Part model, mm, in its own coordinate system. Round coordinates to 2 decimals unless told otherwise and drop trailing zeros. Write each loop counter-clockwise with the first axis right and the second up, starting at its lowest first coordinate (ties: lowest second). Pieces come first, ordered by that corner, then holes. Notation, with made-up numbers: M 67.5,82 L 100.5,82 A22 cw 100.5,102 Z; hole C 81,83.25 d1. An arc over 180 degrees is marked long. Use a Markdown table: item, result. Add a question column.
1) Wall check: probe 1 along X at (y, z) = (-150, 0.85); probe 2 along X at (y, z) = (-32.5, 0.7); probe 3 along Y at (x, z) = (47.5, 0.5). Give the ranges that are in metal, low to high.
2) Slice it at C-C on x = -55.5. Write the cut outline in (y, z), plus the area to 3 significant figures.
3) Two-plate mould, pull along X, no slides. Class faces 1 (the face through (-42.88, -78.28, 0.99)), 2 (the face through (25.72, -165.49, 0.99)), 3 (the face through (-58.785, -0.875, 0.986)): released by +X, released by -X, zero draft, split by the parting line, or undercut.
4) Slice it at A-A on y = -145.5. Write the cut outline in (x, z), plus the area to 3 significant figures.
5) Slice it at B-B on z = 0.3. Give the number of separate pieces and of enclosed holes in the cut face, plus the area to 3 significant figures.
6) Drop flat-ended pins along their axis: P1, Ø1, axis at y = 27, z = 0.5, coming from the -X side (3 decimals); P2, Ø1.5, axis at x = 59.22, y = 46.85, coming from the -Z side. Give the stop position or say it passes through.
```python
from build123d import *

# Parameters (mm, degrees)
BOSS_EXTRUDE1_DEPTH = 2
SKETCH3_R           = 1.25
F_45_DEGREES_DEPTH  = 188.552659272
SKETCH4_R           = 1.5
CUT_EXTRUDE2_DEPTH  = 188.552659272
FILLET1_R           = 5
FILLET2_R           = 5
FILLET3_R           = 5
FILLET4_R           = 5
FILLET5_R           = 5
FILLET6_R           = 5
FILLET7_R           = 5
FILLET8_R           = 5
FILLET9_R           = 5
FILLET10_R          = 5
FILLET11_R          = 5
FILLET12_R          = 5


with BuildPart() as part:
    # Sketch2 → Boss-Extrude1 (new body)
    with BuildSketch(Plane.XY):
        with BuildLine():
            Line((-79.195959493, 62.225396744), (-62.225396744, 79.195959493))
            ThreePointArc((-62.225396744, 79.195959493), (-44.806778225, 80.702789346), (-30, 90))
            Line((-30, 90), (30, 90))
            ThreePointArc((30, 90), (44.806778225, 80.702789346), (62.225396744, 79.195959493))
            Line((62.225396744, 79.195959493), (79.195959493, 62.225396744))
            ThreePointArc((79.195959493, 62.225396744), (58.781303002, 0), (79.195959493, -62.225396744))
            Line((79.195959493, -62.225396744), (62.225396744, -79.195959493))
            ThreePointArc((62.225396744, -79.195959493), (43.875108319, -77.923881554), (30, -90))
            Line((30, -90), (30, -155))
            ThreePointArc((30, -155), (25.606601718, -165.606601718), (15, -170))
            Line((15, -170), (-15, -170))
            ThreePointArc((-15, -170), (-25.606601718, -165.606601718), (-30, -155))
            Line((-30, -155), (-30, -90))
            ThreePointArc((-30, -90), (-43.875108319, -77.923881554), (-62.225396744, -79.195959493))
            Line((-62.225396744, -79.195959493), (-79.195959493, -62.225396744))
            ThreePointArc((-79.195959493, -62.225396744), (-58.781303002, 0), (-79.195959493, 62.225396744))
        make_face()
    extrude(amount=BOSS_EXTRUDE1_DEPTH)

    # Sketch3 → 45 Degrees (cut, through all)
    with BuildSketch(Plane.XY.offset(2)):
        with Locations((-73.362328548, 60.987959877)):
            Circle(SKETCH3_R)
        with Locations((-59.220192924, 46.845824254)):
            Circle(SKETCH3_R)
        with Locations(Location((-60.987959877, 73.362328548, 0), (0, 0, 180))):
            Circle(SKETCH3_R)
        with Locations(Location((-46.845824254, 59.220192924, 0), (0, 0, 180))):
            Circle(SKETCH3_R)
        with Locations(Location((59.220192924, 46.845824254, 0), (0, 0, 180))):
            Circle(SKETCH3_R)
        with Locations(Location((73.362328548, 60.987959877, 0), (0, 0, 180))):
            Circle(SKETCH3_R)
        with Locations((60.987959877, 73.362328548)):
            Circle(SKETCH3_R)
        with Locations((46.845824254, 59.220192924)):
            Circle(SKETCH3_R)
        with Locations(Location((-59.220192924, -46.845824254, 0), (0, 0, 180))):
            Circle(SKETCH3_R)
        with Locations((-46.845824254, -59.220192924)):
            Circle(SKETCH3_R)
        with Locations((-60.987959877, -73.362328548)):
            Circle(SKETCH3_R)
        with Locations(Location((-73.362328548, -60.987959877, 0), (0, 0, 180))):
            Circle(SKETCH3_R)
        with Locations((59.220192924, -46.845824254)):
            Circle(SKETCH3_R)
        with Locations((73.362328548, -60.987959877)):
            Circle(SKETCH3_R)
        with Locations(Location((60.987959877, -73.362328548, 0), (0, 0, 180))):
            Circle(SKETCH3_R)
        with Locations(Location((46.845824254, -59.220192924, 0), (0, 0, 180))):
            Circle(SKETCH3_R)
    extrude(amount=-F_45_DEGREES_DEPTH, mode=Mode.SUBTRACT)

    # Sketch4 → Cut-Extrude2 (cut, through all)
    with BuildSketch(Plane.XY.offset(2)):
        with Locations((-20.76, -150)):
            Circle(SKETCH4_R)
        with Locations((20, -150)):
            Circle(SKETCH4_R)
        with Locations((-20.76, -74.5)):
            Circle(SKETCH4_R)
        with Locations((20, -74.5)):
            Circle(SKETCH4_R)
    extrude(amount=-CUT_EXTRUDE2_DEPTH, mode=Mode.SUBTRACT)

    # Fillet1
    fillet1_edges = [part.edges().sort_by_distance(p)[0] for p in [
        (-30, -90, 1),
    ]]
    fillet(fillet1_edges, radius=FILLET1_R)

    # Fillet2
    fillet2_edges = [part.edges().sort_by_distance(p)[0] for p in [
        (-62.225396744, -79.195959493, 1),
    ]]
    fillet(fillet2_edges, radius=FILLET2_R)

    # Fillet3
    fillet3_edges = [part.edges().sort_by_distance(p)[0] for p in [
        (30, -90, 1),
    ]]
    fillet(fillet3_edges, radius=FILLET3_R)

    # Fillet4
    fillet4_edges = [part.edges().sort_by_distance(p)[0] for p in [
        (62.225396744, -79.195959493, 1),
    ]]
    fillet(fillet4_edges, radius=FILLET4_R)

    # Fillet5
    fillet5_edges = [part.edges().sort_by_distance(p)[0] for p in [
        (79.195959493, -62.225396744, 1),
    ]]
    fillet(fillet5_edges, radius=FILLET5_R)

    # Fillet6
    fillet6_edges = [part.edges().sort_by_distance(p)[0] for p in [
        (-79.195959493, -62.225396744, 1),
    ]]
    fillet(fillet6_edges, radius=FILLET6_R)

    # Fillet7
    fillet7_edges = [part.edges().sort_by_distance(p)[0] for p in [
        (-79.195959493, 62.225396744, 1),
    ]]
    fillet(fillet7_edges, radius=FILLET7_R)

    # Fillet8
    fillet8_edges = [part.edges().sort_by_distance(p)[0] for p in [
        (-62.225396744, 79.195959493, 1),
    ]]
    fillet(fillet8_edges, radius=FILLET8_R)

    # Fillet9
    fillet9_edges = [part.edges().sort_by_distance(p)[0] for p in [
        (-30, 90, 1),
    ]]
    fillet(fillet9_edges, radius=FILLET9_R)

    # Fillet10
    fillet10_edges = [part.edges().sort_by_distance(p)[0] for p in [
        (30, 90, 1),
    ]]
    fillet(fillet10_edges, radius=FILLET10_R)

    # Fillet11
    fillet11_edges = [part.edges().sort_by_distance(p)[0] for p in [
        (62.225396744, 79.195959493, 1),
    ]]
    fillet(fillet11_edges, radius=FILLET11_R)

    # Fillet12
    fillet12_edges = [part.edges().sort_by_distance(p)[0] for p in [
        (79.195959493, 62.225396744, 1),
    ]]
    fillet(fillet12_edges, radius=FILLET12_R)


solid = part.part
```
Entries:
| question | item | result |
|---|---|---|
| 1 | probe 1 | x = -30 to -22.26, -19.26 to 18.5, 21.5 to 30 |
| 1 | probe 2 | x = -63.94 to 63.94 |
| 1 | probe 3 | y = -77.02 to -60.29, -58.16 to 58.16, 60.29 to 79.91 |
| 2 | outline | M -77.01,0 L 78.79,0 L 78.79,2 L -77.01,2 Z |
| 2 | area | 312 mm^2 |
| 3 | face 1 | undercut |
| 3 | face 2 | released by +X |
| 3 | face 3 | released by -X |
| 4 | outline | M -30,0 L 30,0 L 30,2 L -30,2 Z |
| 4 | area | 120 mm^2 |
| 5 | separate pieces | 1 |
| 5 | enclosed holes | 20 |
| 5 | area | 27,100 mm^2 |
| 6 | P1 | stops at x = -62.445 |
| 6 | P2 | passes through |
